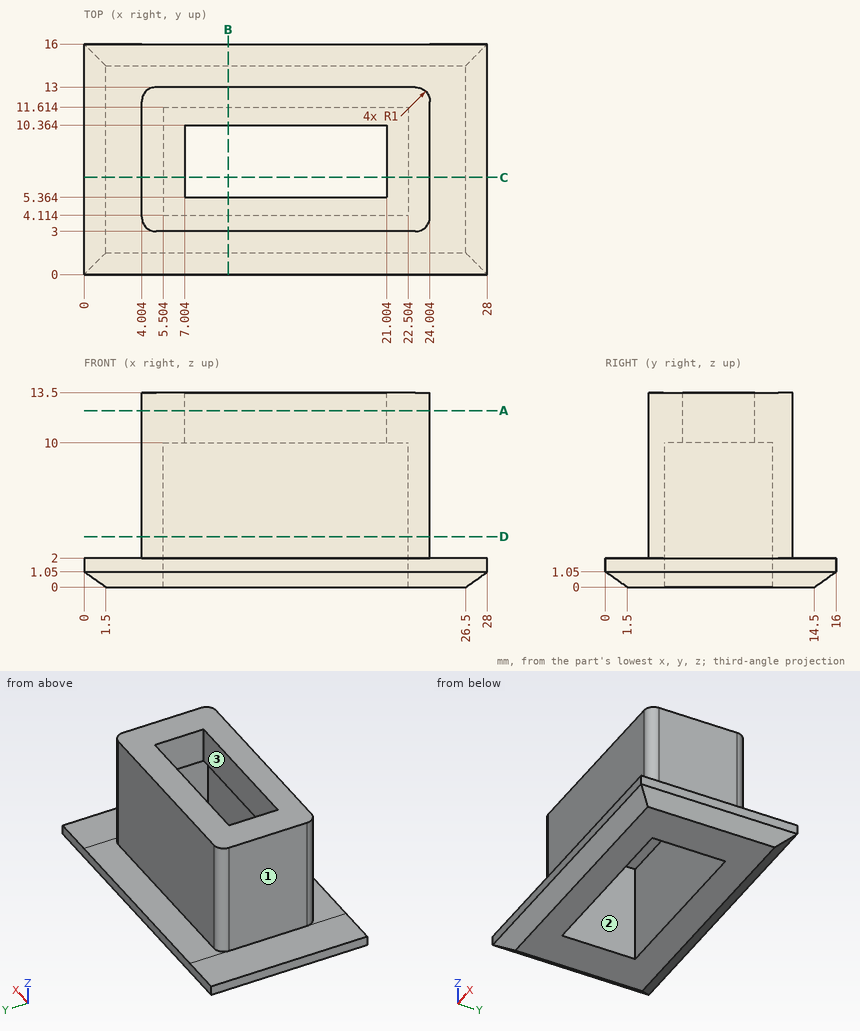
The figure shows three views and two pictorial views of one solid part (mm, origin at its lowest corner). Answer the questions. A direction names the side the tool comes from. Round coordinates to 2 decimals unless told otherwise and drop trailing zeros. Order: outer loops, then holes, each group sorted by start corner. A loop starts at its lowest first (then second) coordinate and runs counter-clockwise, first axis right, second up.
Q1. Find the intervals of material crossed by line 1 along X through (y, z) = (9, 11.5); line 2 along Y through (x, z) = (11.5, 1.5); line 3 along Y through (x, z) = (12.5, 9), in increasing order.
Solution:
line 1: x = 4 to 7, 21 to 24
line 2: y = 0 to 4.11, 11.61 to 16
line 3: y = 3 to 4.11, 11.61 to 13
Q2. A cutting plane is placed at C-C, the plane y = 6.75. Determine the outline of the cut face in (x, z).
Solution:
outline: (0, 1.05) - (1.5, 0) - (5.5, 0) - (5.5, 10) - (7, 10) - (7, 13.5) - (4, 13.5) - (4, 2) - (0, 2) - close; (21, 10) - (22.5, 10) - (22.5, 0) - (26.5, 0) - (28, 1.05) - (28, 2) - (24, 2) - (24, 13.5) - (21, 13.5) - close
Q3. A tool of negligible diameter and unlimited length cuts with its end or side. For the marked faces 1, 2 and 3, from which of +Z, -Z, +X, -X, +Y, -Y can it reach the whole face along a straight path? Write none if from no direction.
Solution:
face 1: +Z, -X, +Y, -Y
face 2: -Z
face 3: +Z, -Z
Q4. A cutting plane is placed at A-A, the plane z = 12.25. Determine the outline of the cut face in (x, y), then the cut area to 3 significant figures.
Solution:
outline: (4, 4) arc R1 ccw to (5, 3) - (23, 3) arc R1 ccw to (24, 4) - (24, 12) arc R1 ccw to (23, 13) - (5, 13) arc R1 ccw to (4, 12) - close; hole (7, 5.36) - (21, 5.36) - (21, 10.36) - (7, 10.36) - close
area: 129 mm2
Q5. A cutting plane is placed at B-B, the plane x = 10. Determine the outline of the cut face in (y, z).
Solution:
outline: (0, 1.05) - (1.5, 0) - (4.11, 0) - (4.11, 10) - (5.36, 10) - (5.36, 13.5) - (3, 13.5) - (3, 2) - (0, 2) - close; (10.36, 10) - (11.61, 10) - (11.61, 0) - (14.5, 0) - (16, 1.05) - (16, 2) - (13, 2) - (13, 13.5) - (10.36, 13.5) - close
Q6. A cutting plane is placed at D-D, the plane z = 3.5. Determine the outline of the cut face in (x, y).
Solution:
outline: (4, 4) arc R1 ccw to (5, 3) - (23, 3) arc R1 ccw to (24, 4) - (24, 12) arc R1 ccw to (23, 13) - (5, 13) arc R1 ccw to (4, 12) - close; hole (5.5, 4.11) - (22.5, 4.11) - (22.5, 11.61) - (5.5, 11.61) - close
Q7. Given pin 1 Ø3 at (x, z) = (18, 3) entering from +Y; pin 2 Ø2 at (y, z) = (3.5, 5.5) entering from -X; pin 3 Ø3 at (x, z) = (11, 11.5) entering from +Y; pin 4 Ø8 at (x, z) = (13, 6.5) entering from -Y, each flat-ended and moving along its own axis, determine where each tip first touches the part or whether it passes through.
Solution:
pin 1: stops at y = 16
pin 2: stops at x = 4
pin 3: stops at y = 13
pin 4: stops at y = 3
